Geometry: final body of the model. Coordinates: model frame, mm. A direction names the side the tool comes from. Give positions to 0.01 mm unless a question says otherwise; leave off trailing zeros. Write each loop counter-clockwise with the first axis right and the second up, starting at its lowest first coordinate (ties: lowest second). Pieces come first, ordered by that corner, then holes. Notation, with made-up numbers: M 89,68 L 120,68 A34 cw 120,106 Z; hole C 89,-28.5 d8. An arc over 180 degrees is marked long. Use a Markdown table: item, result. Add a question column.
1) Set-up query: faces 1 (the cylindrical face through (-75.428, -28.753, -26.497)), 2 (the flat face through (-48.55, 14.78, -14.79)), 3 (the flat face through (-80.875, -11.132, -28.028)). Return all of +Z, -Z, +X, -X, +Y, -Y with unobstructed straight access to the full face (end or side cutting, diameter ignored); none if empty.
2) Section A-A on y = -8. Return the cut outline in (x, z).
3) Line query: line 1 (Y direction, x = -71.7, z = -18); line 2 (Y direction, x = -71.7, z = -22.5); line 3 (Y direction, x = -79.1, z = -18.5). Output: solid intervals per line, ascending.
4) Draft query along X for faces 4 (the flat face through (-76.4, 0, -14.8)), 5 (the cylindrical face through (-109.2, -55.86, -14.79)), 6 (the flat face through (-121.08, 14.72, -14.79)). Return one class per face: +X half, -X half, draft (parallel to the pull), parting line (faces both ways), or undercut.
5) Section B-B on y = -24.5. Return the cut outline in (x, z).
6) Section C-C on z = -19. State how many separate pieces and enclosed holes the cut face has, then the cut area to 3 significant figures.
7) Pin query (flat end, axial travel): pin 1 (3.5 mm diameter, centred on x = -79.1, y = -8, fed in from -Z); pin 2 (2 mm diameter, centred on x = -32, z = -19, fed in from -Y); pin 3 (3.5 mm diameter, centred on y = -31, z = -18, fed in from +X); pin 4 (4.5 mm diameter, centred on y = -37, z = -25, fed in from -X). Return the tip coordinate at first contact, or that it passes through.
```python
from build123d import *

# Parameters (mm, degrees)
RESSALTO_EXTRUS_O1_DEPTH          = 30
RESSALTO_EXTRUS_O2_DEPTH          = 30
ESBO_O3_W                         = 19.4
ESBO_O3_H                         = 3.2
CORTE_EXTRUS_O1_DEPTH             = 23.85
ESBO_O4_W                         = 5.4
ESBO_O4_H                         = 23.8
CORTE_EXTRUS_O2_DEPTH             = 26.5
ESBO_O5_W                         = 19.4
ESBO_O5_H                         = 53
CORTE_EXTRUS_O3_DEPTH             = 15.6
FILETE1_R                         = 5
ESBO_O6_W                         = 69.4
ESBO_O6_H                         = 15.6
CORTE_EXTRUS_O4_DEPTH             = 10
FILETE2_R                         = 3
RESSALTO_EXTRUS_O3_START          = 15.6
RESSALTO_EXTRUS_O3_DEPTH          = 15.6
ESBO_O8_R                         = 1.85
CORTE_EXTRUS_O5_DEPTH             = 165.173688513
CORTE_EXTRUS_O6_DEPTH             = 4
ESBO_O10_W                        = 14.4
ESBO_O10_H                        = 28.961678943
RESSALTO_EXTRUS_O4_DEPTH          = 19.4
RESSALTO_EXTRUS_O5_START          = 15.6
ESBO_O11_R                        = 1.85
RESSALTO_EXTRUS_O5_DEPTH          = 15.6
ESBO_O12_W                        = 35.911027454
ESBO_O12_H                        = 55
CORTE_EXTRUS_O7_DEPTH             = 15
CORTE_EXTRUS_O8_DEPTH             = 2
CORTE_EXTRUS_O8_DEPTH_BACK        = 2
ESBO_O13_R                        = 11.5
CORTE_EXTRUS_O9_REACH             = 104.733
ESBO_O14_R                        = 5.5
CORTE_EXTRUS_O9_DIRECTION_2_REACH = 104.733
CORTE_EXTRUS_O10_DEPTH            = 4


with BuildPart() as part:
    # Esboço1 → Ressalto-extrusão1 (new body)
    with BuildSketch(Plane.XY):
        Polygon((-148.507415706, 17), (-149.671194836, 12.5), (-150.8, 12.5), (-150.8, 0), (0, 0), (0, 12.5), (-1.125252364, 12.5), (-2.289031494, 17), (-3.994153806, 17), (-5.157932936, 12.5), (-7.408437664, 12.5), (-8.572216794, 17), (-10.277339106, 17), (-11.441118236, 12.5), (-13.691622964, 12.5), (-14.855402094, 17), (-16.560524406, 17), (-17.724303536, 12.5), (-19.974808264, 12.5), (-21.138587394, 17), (-22.843709706, 17), (-24.007488836, 12.5), (-26.257993564, 12.5), (-27.421772694, 17), (-29.126895006, 17), (-30.290674136, 12.5), (-32.541178864, 12.5), (-33.704957994, 17), (-35.410080306, 17), (-36.573859436, 12.5), (-38.824364164, 12.5), (-39.988143294, 17), (-41.693265606, 17), (-42.857044736, 12.5), (-45.107549464, 12.5), (-46.271328594, 17), (-47.976450906, 17), (-49.140230036, 12.5), (-51.390734764, 12.5), (-52.554513894, 17), (-54.259636206, 17), (-55.423415336, 12.5), (-57.673920064, 12.5), (-58.837699194, 17), (-60.542821506, 17), (-61.706600636, 12.5), (-63.957105364, 12.5), (-65.120884494, 17), (-66.826006806, 17), (-67.989785936, 12.5), (-70.240290664, 12.5), (-71.404069794, 17), (-73.109192106, 17), (-74.272971236, 12.5), (-76.523475964, 12.5), (-77.687255094, 17), (-79.392377406, 17), (-80.556156536, 12.5), (-82.806661264, 12.5), (-83.970440394, 17), (-85.675562706, 17), (-86.839341836, 12.5), (-89.089846564, 12.5), (-90.253625694, 17), (-91.958748006, 17), (-93.122527136, 12.5), (-95.373031864, 12.5), (-96.536810994, 17), (-98.241933306, 17), (-99.405712436, 12.5), (-101.656217164, 12.5), (-102.819996294, 17), (-104.525118606, 17), (-105.688897736, 12.5), (-107.939402464, 12.5), (-109.103181594, 17), (-110.808303906, 17), (-111.972083036, 12.5), (-114.222587764, 12.5), (-115.386366894, 17), (-117.091489206, 17), (-118.255268336, 12.5), (-120.505773064, 12.5), (-121.669552194, 17), (-123.374674506, 17), (-124.538453636, 12.5), (-126.788958364, 12.5), (-127.952737494, 17), (-129.657859806, 17), (-130.821638936, 12.5), (-133.072143664, 12.5), (-134.235922794, 17), (-135.941045106, 17), (-137.104824236, 12.5), (-139.355328964, 12.5), (-140.519108094, 17), (-142.224230406, 17), (-143.388009536, 12.5), (-145.638514264, 12.5), (-146.802293394, 17), align=None)
    extrude(amount=-RESSALTO_EXTRUS_O1_DEPTH)

    # Esboço2 → Ressalto-extrusão2 (add)
    with BuildSketch(Plane(origin=(0, 0, -30), x_dir=(-1, 0, 0), z_dir=(0, 0, -1))):
        Polygon((85.1, 0), (65.7, 0), (65.7, -55), (40.7, -55), (40.7, -63), (110.1, -63), (110.1, -55), (85.1, -55), align=None)
    extrude(amount=-RESSALTO_EXTRUS_O2_DEPTH)

    # Esboço3 → Corte-extrusão1 (cut)
    with BuildSketch(Plane.XY):
        with Locations((-75.4, -29)):
            Rectangle(ESBO_O3_W, ESBO_O3_H)
    extrude(amount=-CORTE_EXTRUS_O1_DEPTH, mode=Mode.SUBTRACT)

    # Esboço4 → Corte-extrusão2 (cut)
    with BuildSketch(Plane.XY):
        with Locations((-75.4, -29)):
            Rectangle(ESBO_O4_W, ESBO_O4_H)
    extrude(amount=-CORTE_EXTRUS_O2_DEPTH, mode=Mode.SUBTRACT)

    # Esboço5 → Corte-extrusão3 (cut)
    with BuildSketch(Plane.XY):
        with Locations((-75.4, -26.5)):
            Rectangle(ESBO_O5_W, ESBO_O5_H)
    extrude(amount=-CORTE_EXTRUS_O3_DEPTH, mode=Mode.SUBTRACT)

    # Filete1
    filete1_edges = [part.edges().sort_by_distance(p)[0] for p in [
        (-85.1, 0, -22.8),
        (-65.7, 0, -22.8),
    ]]
    fillet(filete1_edges, radius=FILETE1_R)

    # Esboço6 → Corte-extrusão4 (cut)
    with BuildSketch(Plane.XZ.offset(63)):
        with Locations((-75.4, -7.8)):
            Rectangle(ESBO_O6_W, ESBO_O6_H)
    extrude(amount=-CORTE_EXTRUS_O4_DEPTH, mode=Mode.SUBTRACT)

    # Filete2
    filete2_edges = [part.edges().sort_by_distance(p)[0] for p in [
        (0, 0, -15),
        (-150.8, 0, -15),
        (-85.1, -55, -22.8),
        (-110.1, -55, -22.8),
        (-110.1, -63, -22.8),
        (-40.7, -63, -22.8),
        (-40.7, -55, -22.8),
        (-65.7, -55, -22.8),
    ]]
    fillet(filete2_edges, radius=FILETE2_R)

    # Esboço7 → Ressalto-extrusão3 (add)
    with BuildSketch(Plane.XY.offset(-15.6).offset(RESSALTO_EXTRUS_O3_START)):
        with BuildLine():
            Line((-110.1, -58), (-110.1, -60))
            ThreePointArc((-110.1, -60), (-109.221320344, -62.121320344), (-107.1, -63))
            Line((-107.1, -63), (-43.7, -63))
            ThreePointArc((-43.7, -63), (-41.578679656, -62.121320344), (-40.7, -60))
            Line((-40.7, -60), (-40.7, -58))
            ThreePointArc((-40.7, -58), (-41.578679656, -55.878679656), (-43.7, -55))
            Line((-43.7, -55), (-62.7, -55))
            ThreePointArc((-62.7, -55), (-64.821320344, -54.121320344), (-65.7, -52))
            Line((-65.7, -52), (-65.7, -51.6))
            Line((-65.7, -51.6), (-85.1, -51.6))
            Line((-85.1, -51.6), (-85.1, -52))
            ThreePointArc((-85.1, -52), (-85.978679656, -54.121320344), (-88.1, -55))
            Line((-88.1, -55), (-107.1, -55))
            ThreePointArc((-107.1, -55), (-109.221320344, -55.878679656), (-110.1, -58))
        make_face()
    extrude(amount=-RESSALTO_EXTRUS_O3_DEPTH)

    # Esboço8 → Corte-extrusão5 (cut, through all)
    with BuildSketch(Plane.XY.offset(-15.6)):
        with Locations((-79.1, -8)):
            Circle(ESBO_O8_R)
        with Locations((-71.7, -44.6)):
            Circle(ESBO_O8_R)
    extrude(amount=-CORTE_EXTRUS_O5_DEPTH, mode=Mode.SUBTRACT)

    # Esboço9 → Corte-extrusão6 (cut)
    with BuildSketch(Plane(origin=(0, 0, -30), x_dir=(-1, 0, 0), z_dir=(0, 0, -1))):
        Polygon((79.1, -3.843078062), (75.5, -5.921539031), (75.5, -10.078460969), (79.1, -12.156921938), (82.7, -10.078460969), (82.7, -5.921539031), align=None)
        Polygon((71.7, -40.443078062), (68.1, -42.521539031), (68.1, -46.678460969), (71.7, -48.756921938), (75.3, -46.678460969), (75.3, -42.521539031), align=None)
    extrude(amount=-CORTE_EXTRUS_O6_DEPTH, mode=Mode.SUBTRACT)

    # Esboço10 → Ressalto-extrusão4 (add)
    with BuildSketch(Plane(origin=(-65.7, 0, 0), x_dir=(0, 0, -1), z_dir=(1, 0, 0))):
        with Locations((22.8, -27.2404917)):
            Rectangle(ESBO_O10_W, ESBO_O10_H)
    extrude(amount=-RESSALTO_EXTRUS_O4_DEPTH)

    # Esboço11 → Ressalto-extrusão5 (add)
    with BuildSketch(Plane.XY.offset(-15.6).offset(RESSALTO_EXTRUS_O5_START)):
        with BuildLine():
            Line((-90.1, 0), (-60.7, 0))
            ThreePointArc((-60.7, 0), (-64.235533906, -1.464466094), (-65.7, -5))
            Line((-65.7, -5), (-65.7, -51.6))
            Line((-65.7, -51.6), (-85.1, -51.6))
            Line((-85.1, -51.6), (-85.1, -5))
            ThreePointArc((-85.1, -5), (-86.564466094, -1.464466094), (-90.1, 0))
        make_face()
        with Locations((-79.1, -8)):
            Circle(ESBO_O11_R, mode=Mode.SUBTRACT)
        with Locations((-71.7, -44.6)):
            Circle(ESBO_O11_R, mode=Mode.SUBTRACT)
    extrude(amount=-RESSALTO_EXTRUS_O5_DEPTH)

    # Esboço12 → Corte-extrusão7 (cut)
    with BuildSketch(Plane.XY):
        with Locations((-72.144486273, -27.5)):
            Rectangle(ESBO_O12_W, ESBO_O12_H)
    extrude(amount=-CORTE_EXTRUS_O7_DEPTH, mode=Mode.SUBTRACT)

    # Esboço13 → Corte-extrusão8 (cut, two sides: drawn at the far end of the back side and taken through both)
    with BuildSketch(Plane(origin=(-75.4, 0, 0), x_dir=(0, 0, -1), z_dir=(1, 0, 0)).offset(-CORTE_EXTRUS_O8_DEPTH_BACK)):
        with Locations((15, -28.5)):
            Circle(ESBO_O13_R)
    extrude(amount=CORTE_EXTRUS_O8_DEPTH + CORTE_EXTRUS_O8_DEPTH_BACK, mode=Mode.SUBTRACT)

    # Esboço14 → Corte-extrusão9 (cut, up to next)
    with BuildSketch(Plane(origin=(-75.4, 0, 0), x_dir=(0, 0, -1), z_dir=(1, 0, 0)), mode=Mode.PRIVATE) as corte_extrus_o9_sk1:
        with Locations((15, -28.5)):
            Circle(ESBO_O14_R)
    corte_extrus_o9_tool1 = extrude(corte_extrus_o9_sk1.sketch, amount=-CORTE_EXTRUS_O9_REACH, mode=Mode.PRIVATE) & part.part
    add(corte_extrus_o9_tool1.solids().sort_by_distance((-75.4, -28.5, -15))[0], mode=Mode.SUBTRACT)

    # Esboço14 → Corte-extrusão9 direction 2 (cut, up to next)
    with BuildSketch(Plane(origin=(-75.4, 0, 0), x_dir=(0, 0, -1), z_dir=(1, 0, 0)), mode=Mode.PRIVATE) as corte_extrus_o9_direction_2_sk1:
        with Locations((15, -28.5)):
            Circle(ESBO_O14_R)
    corte_extrus_o9_direction_2_tool1 = extrude(corte_extrus_o9_direction_2_sk1.sketch, amount=CORTE_EXTRUS_O9_DIRECTION_2_REACH, mode=Mode.PRIVATE) & part.part
    add(corte_extrus_o9_direction_2_tool1.solids().sort_by_distance((-75.4, -28.5, -15))[0], mode=Mode.SUBTRACT)

    # Esboço15 → Corte-extrusão10 (cut)
    with BuildSketch(Plane(origin=(0, 0, -30), x_dir=(-1, 0, 0), z_dir=(0, 0, -1))):
        Polygon((69.486000671, -41.721331171), (71.7, -40.443078062), (73.913999329, -41.721331171), align=None)
    extrude(amount=-CORTE_EXTRUS_O10_DEPTH, mode=Mode.SUBTRACT)


solid = part.part
```
Found:
| question | item | result |
|---|---|---|
| 1 | face 1 | +Z |
| 1 | face 2 | +Z, -Z, +Y |
| 1 | face 3 | -Z |
| 2 | outline | M -85.1,-30 L -82.7,-30 L -82.7,-26 L -80.95,-26 L -80.95,-15 L -85.1,-15 Z; M -77.25,-26 L -75.5,-26 L -75.5,-30 L -65.7,-30 L -65.7,-15 L -77.25,-15 Z |
| 3 | line 1 | -63 to -46.45, -42.75 to -33.11, -23.89 to 17 |
| 3 | line 2 | -63 to -46.45, -42.75 to 17 |
| 3 | line 3 | -63 to -32.74, -24.26 to -9.85, -6.15 to 17 |
| 4 | face 4 | draft |
| 4 | face 5 | -X half |
| 4 | face 6 | undercut |
| 5 | outline | M -85.1,-30 L -65.7,-30 L -65.7,-18.77 L -73.4,-18.77 L -73.4,-25.78 L -77.4,-25.78 L -77.4,-18.77 L -85.1,-18.77 Z |
| 6 | separate pieces | 2 |
| 6 | enclosed holes | 2 |
| 6 | area | 3,600 mm² |
| 7 | pin 1 | through |
| 7 | pin 2 | y = 0 |
| 7 | pin 3 | x = -65.7 |
| 7 | pin 4 | x = -85.1 |
